Read the model definition and answer for the solid it produces. Units are mm, in the model's axes. Coordinates: 2 decimals unless noted, no trailing zeros. Loops run counter-clockwise (first coordinate to the right, second up) from the corner with the lowest first, then second, coordinate; pieces in that order, holes last. Notation, with made-up numbers: (55, 59) - (92, 59) arc R20 cw to (92, 92) - close; hole circle Ø1 at (56, 28). An arc over 180 degrees is marked (long way). Use one line per item in the form item = value. Start each with the question number.
1) Each of these flat-tipped pins is pushed along its axis until it touches: P1, Ø6, axis at y = -1, z = 9, coming from the -X side; P2, Ø5, axis at x = 0, y = -15.24, coming from the +Z side; P3, Ø10, axis at x = -3, z = 15, coming from the -Y side. Where does it stop, or does it pass through?
2) A cutting plane is placed at A-A (y = 0). Give the vertices of the cut face in (x, z).
3) A cutting plane is placed at C-C (x = 6). Give the vertices of the cut face in (y, z), and give its area (3 significant figures).
4) The mould has two halves that part along X. Classify faces 1 (the face through (0.34, 13.69, 0.53)), 2 (the face through (4, 12, 1.067)), 3 (the face through (-2.7, -12.15, 13.06)), 4 (the face through (10.6, 3.34, 12.52)): released by +X, released by -X, zero draft, split by the parting line, or undercut.
5) A cutting plane is placed at B-B (x = 0). Give the vertices of the cut face in (y, z), and give its area (3 significant figures).
6) A cutting plane is placed at D-D (z = 15.5). Give the vertices of the cut face in (x, y) (1 decimal), and give its area (3 significant figures).
7) Consider line 1 (Y direction, x = 0, z = 0.75); line 2 (Z direction, x = 11, y = -10.5); line 3 (Y direction, x = -8, z = 22.5). Determine where each line is inside the solid, lowest interval first.
from build123d import *

# Parameters (mm, degrees)
SKETCH1_R                    = 17.78
SKETCH1_R_2                  = 11.1125
BOSS_EXTRUDE1_DEPTH          = 25.4
CUT_EXTRUDE1_START           = -24.3332
SKETCH2_OUTSIDE_W            = 48.828
SKETCH2_OUTSIDE_H            = 48.828
SKETCH2_OUTSIDE_R            = 12.446
CUT_EXTRUDE1_DEPTH           = 24.3332
F_1_8_0_125_DIAMETER_HOLE1_D = 3.175


with BuildPart() as part:
    # Sketch1 → Boss-Extrude1 (new body)
    with BuildSketch(Plane.XY):
        Circle(SKETCH1_R)
        Circle(SKETCH1_R_2, mode=Mode.SUBTRACT)
    extrude(amount=BOSS_EXTRUDE1_DEPTH)

    # Sketch2 outside → Cut-Extrude1 (cut)
    with BuildSketch(Plane.XY.offset(25.4).offset(CUT_EXTRUDE1_START)):
        Rectangle(SKETCH2_OUTSIDE_W, SKETCH2_OUTSIDE_H)
        Circle(SKETCH2_OUTSIDE_R, mode=Mode.SUBTRACT)
    extrude(amount=CUT_EXTRUDE1_DEPTH, mode=Mode.SUBTRACT)

    # 1/8 (0.125) Diameter Hole1 (through all)
    with Locations(Plane.XY.offset(1.0668)):
        with Locations((0, 15.24)):
            f_1_8_0_125_diameter_hole1 = Hole(F_1_8_0_125_DIAMETER_HOLE1_D / 2)

    # Mirror1: 1/8 (0.125) Diameter Hole1 across plane
    add(f_1_8_0_125_diameter_hole1.mirror(Plane.ZX), mode=Mode.SUBTRACT)


solid = part.part
Found:
q1.P1 = -12.45
q1.P2 = 1.07
q1.P3 = -12.45
q2.outline = (-17.78, 0) - (-11.11, 0) - (-11.11, 25.4) - (-12.45, 25.4) - (-12.45, 1.07) - (-17.78, 1.07) - close; (11.11, 0) - (17.78, 0) - (17.78, 1.07) - (12.45, 1.07) - (12.45, 25.4) - (11.11, 25.4) - close
q3.outline = (-16.74, 0) - (-9.35, 0) - (-9.35, 25.4) - (-10.9, 25.4) - (-10.9, 1.07) - (-16.74, 1.07) - close; (9.35, 0) - (16.74, 0) - (16.74, 1.07) - (10.9, 1.07) - (10.9, 25.4) - (9.35, 25.4) - close
q3.area = 91.2 mm^2
q4.face_1 = undercut
q4.face_2 = zero draft
q4.face_3 = split by the parting line
q4.face_4 = undercut
q5.outline = (-17.78, 0) - (-16.83, 0) - (-16.83, 1.07) - (-17.78, 1.07) - close; (-13.65, 0) - (-11.11, 0) - (-11.11, 25.4) - (-12.45, 25.4) - (-12.45, 1.07) - (-13.65, 1.07) - close; (11.11, 0) - (13.65, 0) - (13.65, 1.07) - (12.45, 1.07) - (12.45, 25.4) - (11.11, 25.4) - close; (16.83, 0) - (17.78, 0) - (17.78, 1.07) - (16.83, 1.07) - close
q5.area = 72.3 mm^2
q6.outline = circle Ø24.9 at (0, 0); hole circle Ø22.2 at (0, 0)
q6.area = 98.7 mm^2
q7.line_1 = -17.78 to -16.83, -13.65 to -11.11, 11.11 to 13.65, 16.83 to 17.78
q7.line_2 = 0 to 1.07
q7.line_3 = -9.53 to -7.71, 7.71 to 9.53
